Work out the finished part from the listing and answer in its coordinate system (mm). Face numbers are marked on the shaded views. A direction names the side the tool comes from. Coordinates: 2 decimals unless noted, no trailing zeros. Write each loop counter-clockwise with the first axis right and the second up, starting at its lowest first coordinate (ties: lowest second). Pieces come first, ordered by that corner, then holes. Notation, with made-up numbers: (49.25, 8) - (56.25, 8) arc R35 cw to (56.25, 41) - close; hole circle Ø3 at (40.25, -16.75). An arc over 180 degrees is marked (long way). Use a Markdown table: item, result. Add a question column.
(1) Find the intervals of material crossed by line 1 (Z direction, x = -2.5, y = 0); line 2 (Z direction, x = 3, y = 11); line 3 (Y direction, x = -5, z = 96.35), in increasing order. Write a range as from..to.
(2) The part is cut by section C-C, the plane z = 96.35. Give the vertices of the cut face in (x, y).
(3) The part is cut by section D-D, the plane z = 77. Give the vertices of the cut face in (x, y), then the cut area to 3 significant figures.
(4) The part is cut by section A-A, the plane x = 0. Give the vertices of the cut face in (y, z), then the cut area to 3 significant figures.
(5) Given pin 1 Ø1.5 at (y, z) = (-11, 96.5) entering from -X; pin 2 Ø1.5 at (x, z) = (-2, 32) entering from +Y; pin 3 Ø5 at (x, z) = (11.5, 52) entering from +Y, each flat-ended and moving along its own axis, determine where each tip first touches the part or whether it passes through.
(6) The part is cut by section B-B, the plane y = 0. Give the vertices of the cut face in (x, z).
(7) A tool of negligible diameter and unlimited length cuts with its end or side. For the marked faces 1 and 2, from which of +Z, -Z, +X, -X, +Y, -Y can it reach the whole face along a straight path? Write none if from no direction.
Autodesk Inventor part; units mm, degrees
ref_plane "YZ Plane" through (0, 0, 0) normal (1, 0, 0) x (0, 1, 0)
ref_plane "XZ Plane" through (0, 0, 0) normal (0, 1, 0) x (-1, 0, 0)
ref_plane "XY Plane" through (0, 0, 0) normal (0, 0, 1) x (1, 0, 0)
sketch "Sketch1" plane through (0, 0, 0) normal (0, 0, 1) x (1, 0, 0)
  circle A0 centre (0, 0) radius 10
  dimension "d0" = 20
extrude "Extrusion1" add sketch "Sketch1" along normal blind 70
sketch "Sketch2" plane through (0, 0, 70) normal (0, 0, 1) x (1, 0, 0)
  circle A0 centre (0, 0) radius 16
  dimension "d3" = 32
extrude "Extrusion2" add sketch "Sketch2" along normal blind 40
sketch "Sketch3" plane through (0, 0, 0) normal (1, 0, 0) x (0, 1, 0)
  line L0 (16, 70) -> (-16, 70)
  point P0 (0, 0)
  point P1 (0, 96.35)
  dimension "d6" = 26.35
hole "Hole1" at (0, 0, 96.35) direction (-1, 0, 0) diameter 12.7 end through all both
thread "Thread1"
chamfer "Chamfer1" distance 1 angle 45 2 edges at (-16, 0, 110) (-16, 0, 70)
properties part number "CompressionGripAttachment"
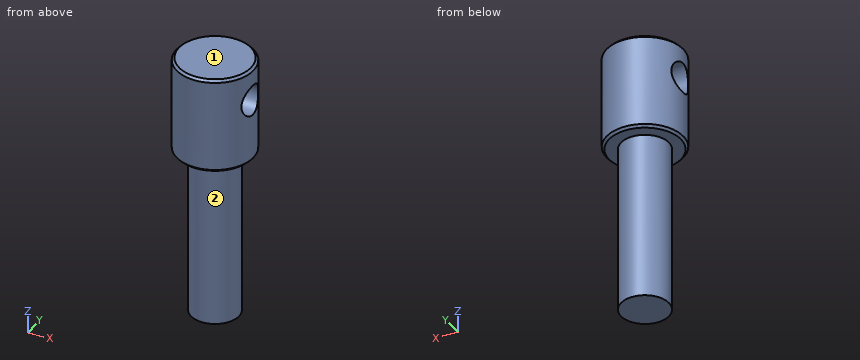
Model answer:
| question | item | result |
|---|---|---|
| 1 | line 1 | 0..90, 102.7..110 |
| 1 | line 2 | 70..110 |
| 1 | line 3 | -15.2..-6.35, 6.35..15.2 |
| 2 | outline | (-14.69, -6.35) arc R16 ccw to (14.69, -6.35) - close; (-14.69, 6.35) - (14.69, 6.35) arc R16 ccw to start |
| 3 | outline | circle Ø32 at (0, 0) |
| 3 | area | 804 mm^2 |
| 4 | outline | (-16, 71) - (-15, 70) - (-10, 70) - (-10, 0) - (10, 0) - (10, 70) - (15, 70) - (16, 71) - (16, 109) - (15, 110) - (-15, 110) - (-16, 109) - close; hole circle Ø12.7 at (0, 96.35) |
| 4 | area | 2,550 mm^2 |
| 5 | pin 1 | x = -12.29 |
| 5 | pin 2 | y = 9.92 |
| 5 | pin 3 | y = 4.36 |
| 6 | outline | (-16, 71) - (-15, 70) - (-10, 70) - (-10, 0) - (10, 0) - (10, 70) - (15, 70) - (16, 71) - (16, 90) - (-16, 90) - close; (-16, 102.7) - (16, 102.7) - (16, 109) - (15, 110) - (-15, 110) - (-16, 109) - close |
| 7 | face 1 | +Z, +X, -X, +Y, -Y |
| 7 | face 2 | -Z |
